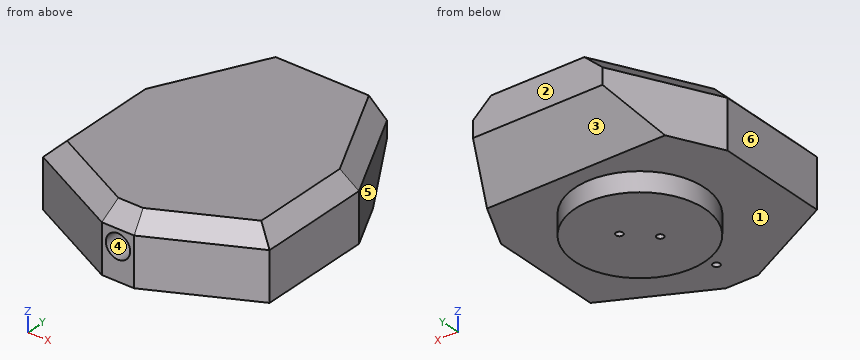
```python
from build123d import *

# Parameters (mm, degrees)
F0_W      = 88.9
F0_H      = 25.4
F1_DEPTH  = 50.8
F3_DEPTH  = 25.4
F5_DEPTH  = 44.451
F6_DEPTH  = 44.451
F7_SIZE   = 6.35
F8_R      = 25.4
F9_DEPTH  = 7.62
F10_R     = 1.35255
F11_DEPTH = 25.4
F12_R     = 4.7625
F13_DEPTH = 19.05
F14_R     = 1.35255
F15_DEPTH = 12.7


with BuildPart() as f1:
    # F0 (on Front) → F1 (new body, symmetric)
    with BuildSketch(Plane.XZ):
        Rectangle(F0_W, F0_H)
    extrude(amount=F1_DEPTH, both=True)

    # F2 (on face) → F3 (cut)
    with BuildSketch(Plane.XY.offset(12.7)):
        Polygon((44.45, -31.75), (6.35, -50.8), (44.45, -50.8), align=None)
        Polygon((-6.35, -50.8), (-44.45, -31.75), (-44.45, -50.8), align=None)
        Polygon((-25.4, 50.8), (-44.45, 50.8), (-44.45, 12.7), align=None)
        Polygon((44.45, 12.7), (44.45, 50.8), (25.4, 50.8), align=None)
    extrude(amount=-F3_DEPTH, mode=Mode.SUBTRACT)

    # F4 (on Right) → F5 (cut, through all)
    with BuildSketch(Plane.YZ):
        Polygon((50.8, 0), (31.75, -12.7), (50.8, -12.7), align=None)
    extrude(amount=-F5_DEPTH, mode=Mode.SUBTRACT)

    # F5_face (on face) → F6 (cut, through all)
    with BuildSketch(Plane(origin=(0, 44.45, -8.466667), x_dir=(0, 1, 0), z_dir=(-1, 0, 0))):
        Polygon((-12.7, 4.233333), (6.35, -8.466667), (6.35, 4.233333), align=None)
    extrude(amount=-F6_DEPTH, mode=Mode.SUBTRACT)

    # F7
    f7_edges = [f1.edges().sort_by_distance(p)[0] for p in [
        (25.4, -41.275, 12.7),
        (0, -50.8, 12.7),
        (-25.4, -41.275, 12.7),
        (-44.45, -9.525, 12.7),
        (-34.925, 31.75, 12.7),
        (44.45, -9.525, 12.7),
        (34.925, 31.75, 12.7),
    ]]
    chamfer(f7_edges, length=F7_SIZE)

    # F8 (on face) → F9 (join)
    with BuildSketch(Plane(origin=(0, 0, -12.7), x_dir=(1, 0, 0), z_dir=(0, 0, -1))):
        Circle(F8_R)
    extrude(amount=F9_DEPTH)

    # F10 (on face) → F11 (cut)
    with BuildSketch(Plane(origin=(0, 0, -20.32), x_dir=(1, 0, 0), z_dir=(0, 0, -1))):
        with Locations((4.490128, -4.490128)):
            Circle(F10_R)
        with Locations((-4.490128, 4.490128)):
            Circle(F10_R)
    extrude(amount=-F11_DEPTH, mode=Mode.SUBTRACT)

    # F12 (on face) → F13 (cut)
    with BuildSketch(Plane.XZ.offset(50.8)):
        Circle(F12_R)
    extrude(amount=-F13_DEPTH, mode=Mode.SUBTRACT)

    # F14 (on face) → F15 (cut)
    with BuildSketch(Plane(origin=(0, 0, -12.7), x_dir=(1, 0, 0), z_dir=(0, 0, -1))):
        with Locations((0, 38.1)):
            Circle(F14_R)
    extrude(amount=-F15_DEPTH, mode=Mode.SUBTRACT)


solid = f1.part
```
Design review of the part built by this model. Coordinates are the model's own, in mm. Face numbers are marked on the shaded views. A direction names the side the tool comes from. Round coordinates to 2 decimals unless told otherwise and drop trailing zeros. Write each loop counter-clockwise with the first axis right and the second up, starting at its lowest first coordinate (ties: lowest second). Pieces come first, ordered by that corner, then holes.
Item 1: We need section A-A on x = 0. Write out the cut boundary in (y, z).
Item 2: Clearance check with flat-ended pins moving along their axes: pin 1 Ø1.4 at (x, y) = (5, 4.5) entering from -Z; pin 2 Ø3 at (x, z) = (19, -7.5) entering from -Y (3 decimals); pin 3 Ø3 at (x, y) = (0, -38.1) entering from -Z. State where each tip first meets the part, or that it passes through.
Item 3: For the marked faces 1 and 2, list the 3-axis set-ups (+Z, -Z, +X, -X, +Y, -Y) from which the entire face can be reached by the end or side of a thin tool; tool diameter is ignored.
Item 4: We need section B-B on y = 0. Write out the cut boundary in (x, z), and give its area (3 significant figures).
Item 5: For probe 1 along Y at (x, z) = (0, -10.25) (3 decimals); probe 2 along Z at (x, y) = (-37.5, 1); probe 3 along X at (y, z) = (0.5, -14), list the stretches that pass through material, from the lowest coordinate up.
Item 6: We need section D-D on z = 8. Write out the cut boundary in (x, y), and give its area (3 significant figures).
Item 7: The part is to be moulded in two halves that separate along X. For the marked faces 3, 4, 5 and 6, say which applies: +X half, -X half, draft (parallel to the pull), parting line (faces both ways), or undercut.
Item 8: We need section C-C on z = -2. Write out the cut boundary in (x, y), and give its area (3 significant figures).
Returned:
1. outline: (-50.8, -12.7) - (-39.45, -12.7) - (-39.45, -4.76) - (-50.8, -4.76) - close; (-50.8, 4.76) - (-31.75, 4.76) - (-31.75, -4.76) - (-36.75, -4.76) - (-36.75, -12.7) - (-25.4, -12.7) - (-25.4, -20.32) - (25.4, -20.32) - (25.4, -12.7) - (31.75, -12.7) - (50.8, 0) - (50.8, 12.7) - (-44.45, 12.7) - (-50.8, 6.35) - close
2. pin 1: stops at z = 5.08
2. pin 2: stops at y = -45.225
2. pin 3: stops at z = -12.7
3. face 1: -Z
3. face 2: +Z, -Z, +X, -X, +Y
4. outline: (-44.45, -12.7) - (-25.4, -12.7) - (-25.4, -20.32) - (25.4, -20.32) - (25.4, -12.7) - (44.45, -12.7) - (44.45, 6.35) - (38.1, 12.7) - (-38.1, 12.7) - (-44.45, 6.35) - close
4. area: 2,600 mm2
5. probe 1: y = -50.8 to -39.453, -36.747 to 35.425
5. probe 2: z = -12.7 to 12.7
5. probe 3: x = -25.4 to 25.4
6. outline: (-42.8, -30.73) - (-5.96, -49.15) - (5.96, -49.15) - (42.8, -30.73) - (42.8, 12.31) - (23.56, 50.8) - (-23.56, 50.8) - (-42.8, 12.31) - close
6. area: 7,140 mm2
7. face 3: draft
7. face 4: undercut
7. face 5: +X half
7. face 6: -X half
8. outline: (-44.45, -31.75) - (-6.35, -50.8) - (-4.32, -50.8) - (-4.32, -31.75) - (4.32, -31.75) - (4.32, -50.8) - (6.35, -50.8) - (44.45, -31.75) - (44.45, 12.7) - (26.9, 47.8) - (-26.9, 47.8) - (-44.45, 12.7) - close; hole circle Ø2.71 at (-4.49, -4.49); hole circle Ø2.71 at (4.49, 4.49)
8. area: 7,250 mm2
